For this review, take the finished solid that the model builds, in its own axes (mm). Face numbers are marked on the shaded views. A direction names the side the tool comes from. Give positions to 0.01 mm unless a question says otherwise; leave off trailing zeros. Order: outer loops, then holes, each group sorted by start corner. A loop starts at its lowest first (then second) coordinate and runs counter-clockwise, first axis right, second up. Notation, with made-up numbers: M 24,-25.75 L 60,-25.75 A14 ccw 60,-20.75 Z; hole C 48,63 d4. An arc over 180 degrees is marked long. Use CSV: the item, a comma, the result in double quotes. Start each with the question number.
(1) Consider section D-D (z = 3.5). Give the number of separate pieces and of enclosed holes in the cut face, and give its area (3 significant figures).
(2) Consider section B-B (y = 6.25). Write out the cut boundary in (x, z).
(3) Clearance check with flat-ended pins moving along their axes: P1, Ø3.5, axis at y = 34, z = 2, coming from the +X side; P2, Ø3.5, axis at x = 69.5, z = 4, coming from the -Y side; P3, Ø1, axis at y = 25.5, z = 3.5, coming from the -X side. State where each tip first meets the part, or that it passes through.
(4) Consider section C-C (x = 9.5). Write out the cut boundary in (y, z), and give its area (3 significant figures).
(5) Consider section A-A (x = 56.5). Write out the cut boundary in (y, z).
(6) Tool access review of the marked faces 3 and 4: name each direction out of +Z, -Z, +X, -X, +Y, -Y from which nothing blocks a thin tool from reaching the whole face with its end or side.
(7) Wall thickness on L1, parallel to Y at x = 19.5, z = 2.25; L2, parallel to Y at x = 29, z = 6; L3, parallel to X at y = 32.5, z = 2: over which ranges is each line inside the solid? List them lowest first. Write a range as from..to.
(8) Draft analysis for pull direction Y (two halves, no side actions). For the marked faces 1 and 2, state which applies: pulls with the +Y half, pulls with the -Y half, needs draft (parallel to the pull), parting line crosses it, or undercut.
Autodesk Inventor part; units mm, degrees
ref_plane "YZ Plane" through (0, 0, 0) normal (1, 0, 0) x (0, 1, 0)
ref_plane "XZ Plane" through (0, 0, 0) normal (0, 1, 0) x (-1, 0, 0)
ref_plane "XY Plane" through (0, 0, 0) normal (0, 0, 1) x (1, 0, 0)
sketch "Sketch1" plane through (0, 0, 0) normal (0, 0, 1) x (1, 0, 0)
  line L0 (0, 0) -> (67.3, 0)
  line L1 (67.3, 0) -> (67.3, 55.5)
  line L2 (67.3, 55.5) -> (0, 55.5)
  line L3 (0, 55.5) -> (0, 0)
  line L4 (7, 48.5) -> (38, 48.5) construction
  line L5 (38, 48.5) -> (38, 17.5) construction
  line L6 (38, 17.5) -> (7, 17.5) construction
  line L7 (7, 17.5) -> (7, 48.5) construction
  line L8 (7, 48.5) -> (17, 48.5) construction
  line L9 (7, 50.1) -> (17, 50.1)
  line L10 (17, 46.9) -> (7, 46.9)
  arc A0 (7, 50.1) -> (7, 46.9) centre (7, 48.5) ccw
  arc A1 (17, 46.9) -> (17, 50.1) centre (17, 48.5) ccw
  line L11 (7, 17.5) -> (17, 17.5) construction
  line L12 (7, 19.1) -> (17, 19.1)
  line L13 (17, 15.9) -> (7, 15.9)
  arc A2 (7, 19.1) -> (7, 15.9) centre (7, 17.5) ccw
  arc A3 (17, 15.9) -> (17, 19.1) centre (17, 17.5) ccw
  line L14 (38, 48.5) -> (48, 48.5) construction
  line L15 (38, 46.9) -> (48, 46.9)
  line L16 (48, 50.1) -> (38, 50.1)
  arc A4 (38, 50.1) -> (38, 46.9) centre (38, 48.5) ccw
  arc A5 (48, 46.9) -> (48, 50.1) centre (48, 48.5) ccw
  line L17 (38, 17.5) -> (48, 17.5) construction
  line L18 (38, 19.1) -> (48, 19.1)
  line L19 (48, 15.9) -> (38, 15.9)
  arc A6 (38, 19.1) -> (38, 15.9) centre (38, 17.5) ccw
  arc A7 (48, 15.9) -> (48, 19.1) centre (48, 17.5) ccw
  line L20 (22.5, 33) -> (32.5, 33) construction
  line L21 (22.5, 44.5) -> (32.5, 44.5)
  line L22 (32.5, 21.5) -> (22.5, 21.5)
  arc A8 (22.5, 44.5) -> (22.5, 21.5) centre (22.5, 33) ccw
  arc A9 (32.5, 21.5) -> (32.5, 44.5) centre (32.5, 33) ccw
  point P0 (12, 48.5)
  point P1 (12, 17.5)
  point P2 (43, 48.5)
  point P3 (43, 17.5)
  point P4 (27.5, 33)
  point P5 (22.5, 48.5)
  point P6 (7, 33)
  dimension "d0" = 31
  dimension "d2" = 10
  dimension "d3" = 3.2
  dimension "d4" = 10
  dimension "d5" = 23
  dimension "d6" = 7
  dimension "d7" = 7
  dimension "d8" = 17.5
  dimension "d9" = 34.8
extrude "Extrusion1" add sketch "Sketch1" along normal blind 6.5
sketch "Sketch2" plane through (0, 0, 6.5) normal (0, 0, 1) x (1, 0, 0)
  line L0 (0, 0) -> (67.3, 0)
  line L1 (0, 55.5) -> (0, 0)
  line L2 (4, 9.5) -> (12, 9.5)
  line L3 (12, 9.5) -> (12, 3)
  line L4 (12, 3) -> (4, 3)
  line L5 (4, 3) -> (4, 9.5)
  line L6 (27, 9.5) -> (35, 9.5)
  line L7 (35, 9.5) -> (35, 3)
  line L8 (35, 3) -> (27, 3)
  line L9 (27, 3) -> (27, 9.5)
  line L10 (12, 3) -> (27, 9.5) construction
  line L11 (27, 3) -> (12, 9.5) construction
  circle A0 centre (19.5, 6.25) radius 2.25
  dimension "d12" = 8
  dimension "d13" = 6.5
  dimension "d14" = 15
  dimension "d15" = 4.5
  dimension "d16" = 3
  dimension "d17" = 4
  dimension "d18" = 8
extrude "Extrusion2" cut sketch "Sketch2" against normal through all
sketch "Sketch3" plane through (0, 0, 6.5) normal (0, 0, 1) x (1, 0, 0)
  arc A0 (32.5, 21.5) -> (32.5, 44.5) centre (32.5, 33) ccw
  line L0 (67.3, 0) -> (67.3, 55.5)
  line L1 (67.3, 35.25) -> (67.3, 30.75)
  line L2 (51, 30.75) -> (51, 35.25)
  line L3 (55, 37.75) -> (62.3, 37.75)
  line L4 (62.3, 28.25) -> (55, 28.25)
  line L5 (51, 35.25) -> (55, 35.25)
  line L6 (62.3, 35.25) -> (67.3, 35.25)
  line L7 (67.3, 30.75) -> (62.3, 30.75)
  line L8 (55, 30.75) -> (51, 30.75)
  line L9 (55, 28.25) -> (55, 30.75)
  line L10 (55, 35.25) -> (55, 37.75)
  line L11 (62.3, 37.75) -> (62.3, 35.25)
  line L12 (62.3, 30.75) -> (62.3, 28.25)
  point P0 (51, 33)
  dimension "d21" = 4.5
  dimension "d22" = 4
  dimension "d23" = 5
  dimension "d24" = 7.3
  dimension "d25" = 2.5
  dimension "d26" = 2.5
extrude "Extrusion3" cut sketch "Sketch3" against normal through all
sketch "Sketch4" plane through (0, 0, 6.5) normal (0, 0, 1) x (1, 0, 0)
  line L0 (67.3, 35.25) -> (67.3, 55.5)
  line L1 (67.3, 0) -> (67.3, 30.75)
  line L2 (51, 30.75) -> (51, 35.25)
  line L3 (67.3, 40.5) -> (71.8, 40.5)
  line L4 (73.8, 42.5) -> (73.8, 46.5)
  line L5 (71.8, 48.5) -> (67.3, 48.5)
  line L6 (67.3, 48.5) -> (67.3, 40.5)
  line L7 (67.3, 25.5) -> (71.8, 25.5)
  line L8 (73.8, 23.5) -> (73.8, 19.5)
  line L9 (71.8, 17.5) -> (67.3, 17.5)
  line L10 (67.3, 17.5) -> (67.3, 25.5)
  arc A0 (73.8, 46.5) -> (71.8, 48.5) centre (71.8, 46.5) ccw
  arc A1 (71.8, 40.5) -> (73.8, 42.5) centre (71.8, 42.5) ccw
  arc A2 (73.8, 23.5) -> (71.8, 25.5) centre (71.8, 23.5) ccw
  arc A3 (71.8, 17.5) -> (73.8, 19.5) centre (71.8, 19.5) ccw
  point P0 (51, 33)
  dimension "d29" = 2
  dimension "d30" = 8
  dimension "d31" = 8
  dimension "d32" = 6.5
  dimension "d33" = 15
  dimension "d34" = 7.5
extrude "Extrusion4" add sketch "Sketch4" against normal blind 6.5
chamfer "Chamfer1" distance 2 angle 45 1 edges at (0, 55.5, 3.25)
sketch "Sketch5" plane through (0, 0, 6.5) normal (0, 0, 1) x (1, 0, 0)
  line L0 (7, 50.1) -> (17, 50.1)
  line L1 (-20.7, -32.99) -> (67.3, -32.99)
  line L2 (67.3, -32.99) -> (67.3, 0)
  line L3 (0, 0) -> (67.3, 0)
  line L4 (-20.7, -32.99) -> (-20.7, -27.99)
  line L5 (-20.7, -27.99) -> (0, 0)
  point P0 (67.3, 55.5)
  dimension "d40" = 88.49
  dimension "d41" = 88
  dimension "d42" = 5
extrude "Extrusion5" add sketch "Sketch5" against normal blind 6.5
sketch "Sketch6" plane through (0, 0, 6.5) normal (0, 0, 1) x (1, 0, 0)
  line L0 (-20.7, -32.99) -> (67.3, -32.99)
  line L1 (-2.25, -16.69) -> (2.25, -16.69)
  line L2 (2.25, -32.99) -> (-2.25, -32.99)
  line L3 (4.75, -20.69) -> (4.75, -27.99)
  line L4 (-4.75, -27.99) -> (-4.75, -20.69)
  line L5 (-4.75, -20.69) -> (-2.25, -20.69)
  line L6 (2.25, -20.69) -> (4.75, -20.69)
  line L7 (4.75, -27.99) -> (2.25, -27.99)
  line L8 (-2.25, -27.99) -> (-4.75, -27.99)
  line L9 (-2.25, -32.99) -> (-2.25, -27.99)
  line L10 (-2.25, -20.69) -> (-2.25, -16.69)
  line L11 (2.25, -16.69) -> (2.25, -20.69)
  line L12 (2.25, -27.99) -> (2.25, -32.99)
  point P0 (0, 0)
  point P1 (0, -16.69)
  dimension "d45" = 4.5
  dimension "d46" = 2.5
  dimension "d47" = 2.5
  dimension "d48" = 5
  dimension "d49" = 4
  dimension "d50" = 7.3
extrude "Extrusion6" cut sketch "Sketch6" against normal through all
properties part number "y_motor_mount" material "Plywood, Finish"
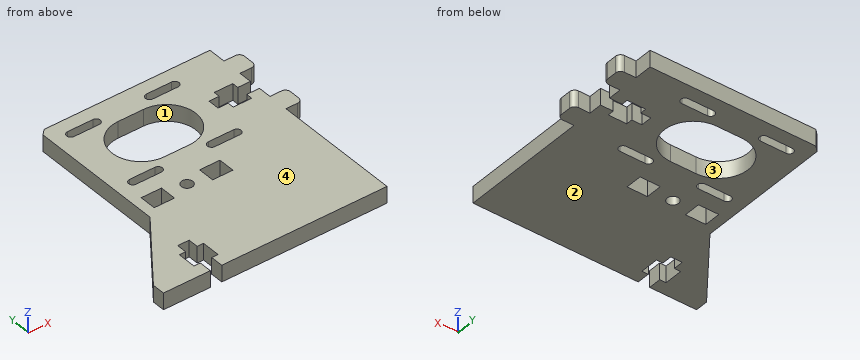
Check result:
1,separate pieces,"1"
1,enclosed holes,"8"
1,area,"5,300 mm^2"
2,outline,"M 0,0 L 4,0 L 4,6.5 L 0,6.5 Z; M 12,0 L 17.25,0 L 17.25,6.5 L 12,6.5 Z; M 21.75,0 L 27,0 L 27,6.5 L 21.75,6.5 Z; M 35,0 L 67.3,0 L 67.3,6.5 L 35,6.5 Z"
3,P1,"stops at x = 67.3"
3,P2,"stops at y = 17.5"
3,P3,"stops at x = 0"
4,outline,"M -32.99,0 L 3,0 L 3,6.5 L -32.99,6.5 Z; M 9.5,0 L 15.9,0 L 15.9,6.5 L 9.5,6.5 Z; M 19.1,0 L 46.9,0 L 46.9,6.5 L 19.1,6.5 Z; M 50.1,0 L 55.5,0 L 55.5,6.5 L 50.1,6.5 Z"
4,area,"491 mm^2"
5,outline,"M -32.99,0 L 28.25,0 L 28.25,6.5 L -32.99,6.5 Z; M 37.75,0 L 55.5,0 L 55.5,6.5 L 37.75,6.5 Z"
6,face 3,"+Z, -Z"
6,face 4,"+Z, +X, -X, +Y, -Y"
7,L1,"y = -32.99..4, 8.5..21.9, 44.1..55.5"
7,L2,"y = -32.99..3, 9.5..21.5, 44.5..55.5"
7,L3,"x = 0..11.01, 43.99..51"
8,face 1,"undercut"
8,face 2,"needs draft"
